from build123d import *

# Parameters (mm, degrees)
SKETCH1_W           = 110.237040332
SKETCH1_H           = 78.14500721
BOSS_EXTRUDE1_DEPTH = 25.4
SKETCH2_R           = 31.75
CUT_EXTRUDE1_DEPTH  = 73.179441694
CHAMFER1_SIZE       = 25.4


with BuildPart() as part:
    # Sketch1 → Boss-Extrude1 (new body)
    with BuildSketch(Plane.XY):
        Rectangle(SKETCH1_W, SKETCH1_H)
    extrude(amount=-BOSS_EXTRUDE1_DEPTH)

    # Sketch2 → Cut-Extrude1 (cut, through all)
    with BuildSketch(Plane.XY):
        Circle(SKETCH2_R)
    extrude(amount=-CUT_EXTRUDE1_DEPTH, mode=Mode.SUBTRACT)

    # Chamfer1
    chamfer1_edges = [part.edges().sort_by_distance(p)[0] for p in [
        (55.118520166, -39.072503605, -12.7),
        (-55.118520166, -39.072503605, -12.7),
        (-55.118520166, 39.072503605, -12.7),
        (55.118520166, 39.072503605, -12.7),
    ]]
    chamfer(chamfer1_edges, length=CHAMFER1_SIZE)


solid = part.part
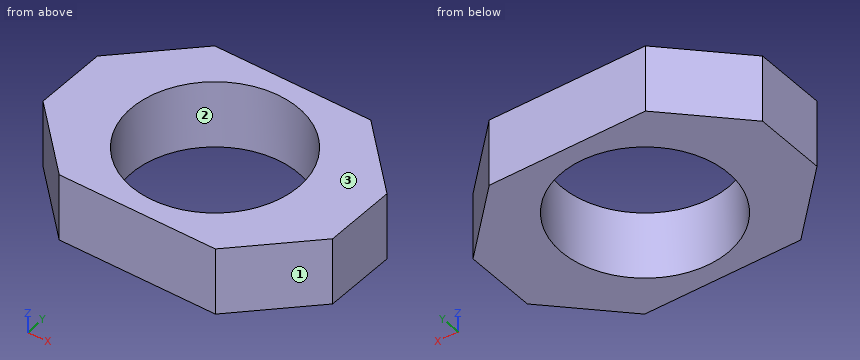
Design review of the part built by this model. Coordinates are the model's own, in mm. Face numbers are marked on the shaded views. Round coordinates to 2 decimals unless told otherwise and drop trailing zeros. Loops run counter-clockwise (first coordinate to the right, second up) from the corner with the lowest first, then second, coordinate; pieces in that order, holes last. Notation, with made-up numbers: (-39.75, 7) -> (-18.75, 7) arc R13 ccw to (-18.75, 22) -> close; hole circle Ø7 at (-9.75, -10.75). An arc over 180 degrees is marked (long way). Use one line per item in the form item = value. Start each with the question number.
Q1. We need section C-C on z = -5.5. Give the boundary of the cut face in (x, y), then the cut area to 3 significant figures.
Q2. We need section A-A on y = -5.5. Give the boundary of the cut face in (x, z), then the cut area to 3 significant figures.
Q3. We need section B-B on x = 0. Give the boundary of the cut face in (y, z), then the cut area to 3 significant figures.
Q4. For pin 1 Ø5 at (x, y) = (-17, -24.5) entering from -Z, flat-tipped, find the tip position at first contact; note if it passes through.
Q5. Wall thickness on line 1 along Y through (x, z) = (0, -14); line 2 along Y through (x, z) = (28, -10.5); line 3 along X through (y, z) = (4, -1.5): over which ranges is each line inside the solid? List them lowest first. Write a range as [from, to].
Q6. We need section D-D on x = 38. Give the boundary of the cut face in (y, z), then the cut area to 3 significant figures.
Q7. Draft analysis for pull direction X (two halves, no side actions). For the marked faces 1, 2 and 3, state which applies: +X half, -X half, draft (parallel to the pull), parting line (faces both ways), or undercut.
Calculated:
q1.outline = (-55.12, -13.67) -> (-29.72, -39.07) -> (29.72, -39.07) -> (55.12, -13.67) -> (55.12, 13.67) -> (29.72, 39.07) -> (-29.72, 39.07) -> (-55.12, 13.67) -> close; hole circle Ø63.5 at (0, 0)
q1.area = 4,160 mm²
q2.outline = (-55.12, -25.4) -> (-31.27, -25.4) -> (-31.27, 0) -> (-55.12, 0) -> close; (31.27, -25.4) -> (55.12, -25.4) -> (55.12, 0) -> (31.27, 0) -> close
q2.area = 1,210 mm²
q3.outline = (-39.07, -25.4) -> (-31.75, -25.4) -> (-31.75, 0) -> (-39.07, 0) -> close; (31.75, -25.4) -> (39.07, -25.4) -> (39.07, 0) -> (31.75, 0) -> close
q3.area = 372 mm²
q4.pin_1 = -25.4
q5.line_1 = [-39.07, -31.75], [31.75, 39.07]
q5.line_2 = [-39.07, -14.97], [14.97, 39.07]
q5.line_3 = [-55.12, -31.5], [31.5, 55.12]
q6.outline = (-30.79, -25.4) -> (30.79, -25.4) -> (30.79, 0) -> (-30.79, 0) -> close
q6.area = 1,560 mm²
q7.face_1 = +X half
q7.face_2 = undercut
q7.face_3 = draft
